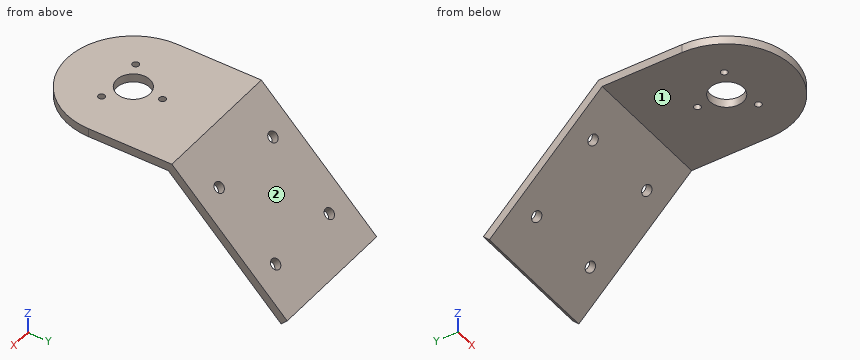
from build123d import *

# Parameters (mm, degrees)
SKETCH1_R           = 6.273243026
SKETCH1_R_2         = 1.25
BOSS_EXTRUDE1_DEPTH = 3.2
BOSS_EXTRUDE2_DEPTH = 50
CUT_EXTRUDE1_REACH  = 74.091
SKETCH3_R           = 2


with BuildPart() as part:
    # Sketch1 → Boss-Extrude1 (new body)
    with BuildSketch(Plane.XY):
        with BuildLine():
            Line((-25, 0), (-25, 30))
            Line((-25, 30), (25, 30))
            Line((25, 30), (25, 0))
            ThreePointArc((25, 0), (0, -25), (-25, 0))
        make_face()
        Circle(SKETCH1_R, mode=Mode.SUBTRACT)
        with Locations((0, 11)):
            Circle(SKETCH1_R_2, mode=Mode.SUBTRACT)
        with Locations((9.526279442, -5.5)):
            Circle(SKETCH1_R_2, mode=Mode.SUBTRACT)
        with Locations((-9.526279442, -5.5)):
            Circle(SKETCH1_R_2, mode=Mode.SUBTRACT)
    extrude(amount=BOSS_EXTRUDE1_DEPTH)

    # Sketch2 → Boss-Extrude2 (add)
    with BuildSketch(Plane(origin=(25, 0, 0), x_dir=(0, 0, -1), z_dir=(1, 0, 0))):
        Polygon((0, 30), (42.426406871, 72.426406871), (40.163665171, 74.689148571), (-3.2, 31.3254834), (-3.2, 30), align=None)
    extrude(amount=-BOSS_EXTRUDE2_DEPTH)

    # Sketch3 → Cut-Extrude1 (cut, up to next)
    with BuildSketch(Plane(origin=(0, 17.2627417, 17.2627417), x_dir=(1, 0, 0), z_dir=(0, 0.707106781, 0.707106781)), mode=Mode.PRIVATE) as cut_extrude1_sk1:
        with Locations((15, 65.550461736)):
            Circle(SKETCH3_R)
    cut_extrude1_tool1 = extrude(cut_extrude1_sk1.sketch, amount=-CUT_EXTRUDE1_REACH, mode=Mode.PRIVATE) & part.part
    add(cut_extrude1_tool1.solids().sort_by_distance((15, 63.613918, -29.088434))[0], mode=Mode.SUBTRACT)
    # Sketch3 → Cut-Extrude1 (cut, up to next)
    with BuildSketch(Plane(origin=(0, 17.2627417, 17.2627417), x_dir=(1, 0, 0), z_dir=(0, 0.707106781, 0.707106781)), mode=Mode.PRIVATE) as cut_extrude1_sk2:
        with Locations((15, 35.550461736)):
            Circle(SKETCH3_R)
    cut_extrude1_tool2 = extrude(cut_extrude1_sk2.sketch, amount=-CUT_EXTRUDE1_REACH, mode=Mode.PRIVATE) & part.part
    add(cut_extrude1_tool2.solids().sort_by_distance((15, 42.400714, -7.875231))[0], mode=Mode.SUBTRACT)
    # Sketch3 → Cut-Extrude1 (cut, up to next)
    with BuildSketch(Plane(origin=(0, 17.2627417, 17.2627417), x_dir=(1, 0, 0), z_dir=(0, 0.707106781, 0.707106781)), mode=Mode.PRIVATE) as cut_extrude1_sk3:
        with Locations((-15, 65.550461736)):
            Circle(SKETCH3_R)
    cut_extrude1_tool3 = extrude(cut_extrude1_sk3.sketch, amount=-CUT_EXTRUDE1_REACH, mode=Mode.PRIVATE) & part.part
    add(cut_extrude1_tool3.solids().sort_by_distance((-15, 63.613918, -29.088434))[0], mode=Mode.SUBTRACT)
    # Sketch3 → Cut-Extrude1 (cut, up to next)
    with BuildSketch(Plane(origin=(0, 17.2627417, 17.2627417), x_dir=(1, 0, 0), z_dir=(0, 0.707106781, 0.707106781)), mode=Mode.PRIVATE) as cut_extrude1_sk4:
        with Locations((-15, 35.550461736)):
            Circle(SKETCH3_R)
    cut_extrude1_tool4 = extrude(cut_extrude1_sk4.sketch, amount=-CUT_EXTRUDE1_REACH, mode=Mode.PRIVATE) & part.part
    add(cut_extrude1_tool4.solids().sort_by_distance((-15, 42.400714, -7.875231))[0], mode=Mode.SUBTRACT)


solid = part.part
Verification items for the finished model (mm, model axes). Face numbers are marked on the shaded views. Give positions to 0.01 mm unless a question says otherwise; leave off trailing zeros. Write each loop counter-clockwise with the first axis right and the second up, starting at its lowest first coordinate (ties: lowest second). Pieces come first, ordered by that corner, then holes. Notation, with made-up numbers: M -4,-4 L 42,-4 A26 ccw 42,23 Z; hole C 52,37.25 d7. An arc over 180 degrees is marked long. Put each result on its own line as item: value. Start each with the question number.
1. Section check B-B (x = 20). Record the cut outline in (y, z), and give its area (3 significant figures).
2. Section check C-C (x = 9.5). Record the cut outline in (y, z).
3. Go/stop test with flat-tipped pins: pin 1 Ø25 at (x, y) = (3, 1) entering from -Z; pin 2 Ø2 at (x, z) = (4, -33) entering from +Y; pin 3 Ø16.5 at (x, y) = (0, 0) entering from +Z; pin 4 Ø8 at (x, z) = (-18.5, -16.5) entering from +Y. Record where each tip stops, or that it passes through.
4. Draft check along Z on the marked faces 1 and 2. Enter one of: +Z half, -Z half, draft (parallel to the pull), parting line (faces both ways), or undercut.
5. Section check D-D (y = 25.5). Record the cut outline in (x, z), and give its area (3 significant figures).
6. Section check A-A (x = 0). Record the cut outline in (y, z), and give its area (3 significant figures).
7. Scan lines: line 1 along Y through (x, z) = (0, 1); line 2 along Z through (x, y) = (-0.5, -6.5); line 3 along Y through (x, z) = (0, 2.55). Record each from-to range of solid material in increasing order. Write a range as [from, to].
Answer list:
1. outline: M -15,0 L 30,0 L 72.43,-42.43 L 74.69,-40.16 L 31.33,3.2 L -15,3.2 Z
1. area: 340 mm2
2. outline: M -23.12,0 L -6.75,0 L -6.75,3.2 L -23.12,3.2 Z; M -4.25,0 L 30,0 L 72.43,-42.43 L 74.69,-40.16 L 31.33,3.2 L -4.25,3.2 Z
3. pin 1: z = 0
3. pin 2: y = 68.53
3. pin 3: z = 3.2
3. pin 4: y = 55.03
4. face 1: -Z half
4. face 2: +Z half
5. outline: M -25,0 L 25,0 L 25,3.2 L -25,3.2 Z
5. area: 160 mm2
6. outline: M -25,0 L -6.27,0 L -6.27,3.2 L -25,3.2 Z; M 6.27,0 L 9.75,0 L 9.75,3.2 L 6.27,3.2 Z; M 12.25,0 L 30,0 L 72.43,-42.43 L 74.69,-40.16 L 31.33,3.2 L 12.25,3.2 Z
6. area: 324 mm2
7. line 1: [-25, -6.27], [6.27, 9.75], [12.25, 33.53]
7. line 2: [0, 3.2]
7. line 3: [-25, -6.27], [6.27, 9.75], [12.25, 31.98]
